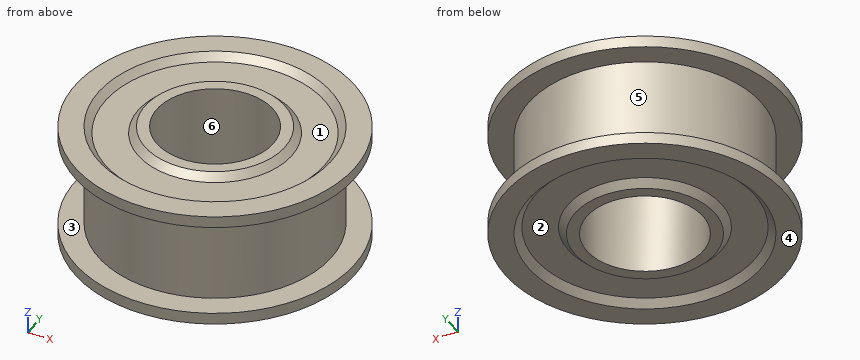
```python
from build123d import *

# Parameters (mm, degrees)
CROQUIS1_R                 = 30
CROQUIS1_R_2               = 12.5
SALIENTE_EXTRUIR1_DEPTH    = 25
CROQUIS3_W                 = 20
CROQUIS3_H                 = 10
CROQUIS4_R                 = 25
CROQUIS4_R_2               = 15
CORTAR_EXTRUIR1_DEPTH      = 1.5
CHAFL_N2_SIZE              = 1.5
CHAFL_N2_OF_SIMETR_A2_SIZE = 1.5


with BuildPart() as part:
    # Croquis1 → Saliente-Extruir1 (new body)
    with BuildSketch(Plane.XY):
        Circle(CROQUIS1_R)
        Circle(CROQUIS1_R_2, mode=Mode.SUBTRACT)
    extrude(amount=SALIENTE_EXTRUIR1_DEPTH)

    # Croquis3 → Cortar-Revolución1 (revolve, cut)
    with BuildSketch(Plane(origin=(0, 0, 0), x_dir=(0, 0, -1), z_dir=(1, 0, 0)), mode=Mode.PRIVATE) as cortar_revoluci_n1_sk:
        with Locations((-12.5, 30)):
            Rectangle(CROQUIS3_W, CROQUIS3_H)
    revolve(cortar_revoluci_n1_sk.sketch.rotate(Axis((0, 0, 25), (0, 0, -1)), 90), axis=Axis((0, 0, 25), (0, 0, -1)), mode=Mode.SUBTRACT)

    # Croquis4 → Cortar-Extruir1 (cut)
    with BuildSketch(Plane.XY.offset(25)):
        Circle(CROQUIS4_R)
        Circle(CROQUIS4_R_2, mode=Mode.SUBTRACT)
    cortar_extruir1 = extrude(amount=-CORTAR_EXTRUIR1_DEPTH, mode=Mode.SUBTRACT)

    # Chaflán2
    chafl_n2_edges = [part.edges().sort_by_distance(p)[0] for p in [
        (-25, 0, 23.5),
        (-15, 0, 23.5),
    ]]
    chamfer(chafl_n2_edges, length=CHAFL_N2_SIZE - 0.0001)  # a hair under: the kernel refuses the full size

    # Simetría2: Cortar-Extruir1 across plane
    add(cortar_extruir1.mirror(Plane.XY.offset(12.5)), mode=Mode.SUBTRACT)

    # Chaflán2 of Simetría2
    chafl_n2_of_simetr_a2_edges = [part.edges().sort_by_distance(p)[0] for p in [
        (-25, 0, 1.5),
        (-15, 0, 1.5),
    ]]
    chamfer(chafl_n2_of_simetr_a2_edges, length=CHAFL_N2_OF_SIMETR_A2_SIZE - 0.0001)  # a hair under: the kernel refuses the full size


solid = part.part
```
The model under review builds one solid part; all positions refer to its coordinate system, in mm. Face numbers are marked on the shaded views. A direction names the side the tool comes from. Coordinates: 2 decimals unless noted, no trailing zeros. Write each loop counter-clockwise with the first axis right and the second up, starting at its lowest first coordinate (ties: lowest second). Pieces come first, ordered by that corner, then holes. Notation, with made-up numbers: (51, -30.75) - (58, -30.75) arc R6 cw to (58, -19.75) - close; hole circle Ø8 at (64, -10). An arc over 180 degrees is marked (long way). Write item = value, one per line.
(1) For line 1 (Z direction, x = -11, y = -27); line 2 (X direction, y = 0.5, z = 14.5) (3 decimals); line 3 (Y direction, x = 10, z = 20), list the stretches that pass through material, from the lowest coordinate up. Write a range as [from, to].
Result sheet:
line_1 = [0, 2.5], [22.5, 25]
line_2 = [-24.995, -12.49], [12.49, 24.995]
line_3 = [-22.91, -7.5], [7.5, 22.91]
(2) For P1, Ø8, axis at x = -21.5, z = 11.5, coming from the +Y side; P2, Ø5, axis at x = 14.5, z = 14.5, coming from the +Y side; P3, Ø4, axis at y = 10.5, z = 9, coming from the -X side, all flat-tipped, find the tip position at first contact; note any pin that passes through.
Result sheet:
P1 = 17.85
P2 = 21.93
P3 = -23.51
(3) Mouldability with a two-part tool opening along Y and no side actions: class the marked faces 4, 5 and 6 as pulls with the +Y half, pulls with the -Y half, needs draft (parallel to the pull), parting line crosses it, or undercut.
Result sheet:
face_4 = needs draft
face_5 = parting line crosses it
face_6 = undercut
(4) Machinability: for the marked faces 1, 2 and 3, which of the approach directions +Z, -Z, +X, -X, +Y, -Y give a long, thin tool a straight path to every point of the face, cutting with its end or side? Answer none if there is none.
Result sheet:
face_1 = +Z
face_2 = -Z
face_3 = none
(5) Consider section A-A, the plane z = 4.25. Give the boundary of the cut face in (x, y).
Result sheet:
outline = circle Ø50 at (0, 0); hole circle Ø25 at (0, 0)
